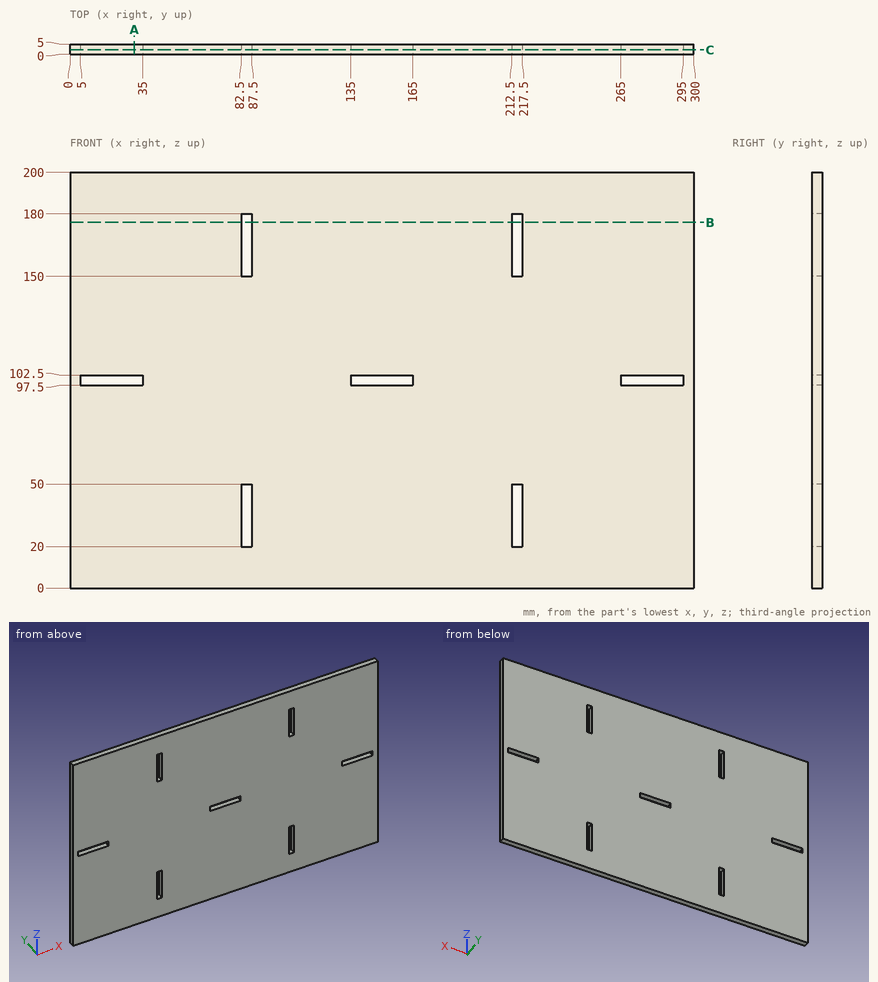
Geometry: see drawing. Coordinates: mm, zero at the bounding-box minimum. Give positions to 0.01 mm unless a question says otherwise; leave off trailing zeros. Loops run counter-clockwise (first coordinate to the right, second up) from the corner with the lowest first, then second, coordinate; pieces in that order, holes last. Notation, with made-up numbers: (39, -0.75) -> (85, -0.75) arc R9 cw to (85, 12.25) -> close; hole circle Ø10 at (12.25, 80). An arc over 180 degrees is marked (long way). Answer as a JSON object with one key per item and string values. Group by question number.
Item 1: Line query: probe 1 along X at (y, z) = (3.45, 36). Output: solid intervals per line, ascending.
Item 2: Cut plane A-A, the plane x = 31. Return the cut outline in (y, z), and give its area (3 significant figures).
Item 3: Pin query (flat end, axial travel): P1, Ø1.5, axis at x = 216, y = 1.5, coming from the -Z side. Return the tip coordinate at first contact, or that it passes through.
Item 4: Cut plane C-C, the plane y = 2.2. State how many separate pieces and enclosed holes the cut face has, and give its area (4 significant figures).
Item 5: Cut plane B-B, the plane z = 176. Return the cut outline in (x, y).
Checks:
{
 "1": {"probe 1": "x = 0 to 82.5, 87.5 to 212.5, 217.5 to 300"},
 "2": {"outline": "(0, 0) -> (5, 0) -> (5, 97.5) -> (0, 97.5) -> close; (0, 102.5) -> (5, 102.5) -> (5, 200) -> (0, 200) -> close", "area": "975 mm²"},
 "3": {"P1": "stops at z = 0"},
 "4": {"separate pieces": "1", "enclosed holes": "7", "area": "58,950 mm²"},
 "5": {"outline": "(0, 0) -> (82.5, 0) -> (82.5, 5) -> (0, 5) -> close; (87.5, 0) -> (212.5, 0) -> (212.5, 5) -> (87.5, 5) -> close; (217.5, 0) -> (300, 0) -> (300, 5) -> (217.5, 5) -> close"}
}
